Read the model definition and answer for the solid it produces. Units are mm, in the model's axes. Coordinates: 2 decimals unless noted, no trailing zeros. Write each loop counter-clockwise with the first axis right and the second up, starting at its lowest first coordinate (ties: lowest second). Pieces come first, ordered by that corner, then holes.
(1) Straight lines are drawn through the part: line 1 along Z through (x, y) = (2.65, 13.25); line 2 along Y through (x, z) = (2.35, -90.5); line 3 along Z through (x, y) = (1.6, 1.5). For each, find the intervals that lie inside material, in ascending order.
(2) The part is cut by section A-A, the plane y = 13.25. Determine the outline of the cut face in (x, z), and give its area (3 significant figures).
(3) The part is cut by section C-C, the plane z = -89.5. Determine the outline of the cut face in (x, y), and give its area (3 significant figures).
(4) The part is cut by section B-B, the plane x = 1.35. Determine the outline of the cut face in (y, z).
(5) Given pin 1 (0.9 mm diameter, centred on x = 2, z = -92.5, fed in from +Y); pin 2 (1.5 mm diameter, centred on x = 2, z = -123, fed in from -Y); pin 3 (1.5 mm diameter, centred on x = 1.5, y = 13.5, fed in from -Z), each flat-ended and moving along its own axis, determine where each tip first touches the part or whether it passes through.
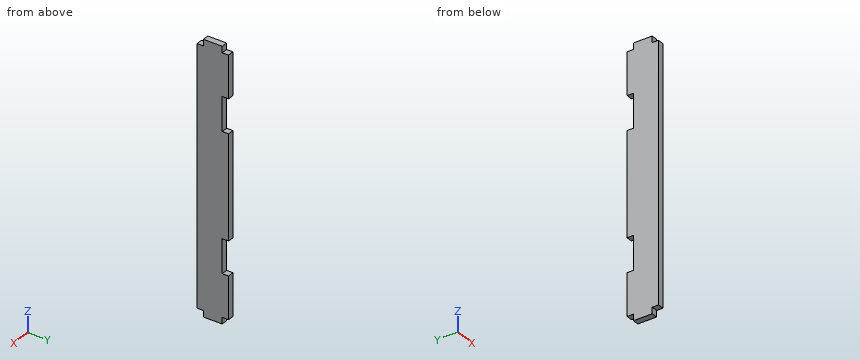
```python
from build123d import *

# Parameters (mm, degrees)
SKETCH1_W           = 3
SKETCH1_H           = 9
BOSS_EXTRUDE1_DEPTH = 3


with BuildPart() as part:
    # Sketch1 → Boss-Extrude1 (new body)
    with BuildSketch(Plane(origin=(0, 0, 0), x_dir=(0, 0, -1), z_dir=(1, 0, 0))):
        Polygon((0, 3), (0, 0), (121, 0), (121, 3), (121, 12), (121, 15), (101, 15), (101, 12), (85, 12), (85, 15), (36, 15), (36, 12), (20, 12), (20, 15), (0, 15), (0, 12), align=None)
        with Locations((-1.5, 7.5)):
            Rectangle(SKETCH1_W, SKETCH1_H)
        with Locations((122.5, 7.5)):
            Rectangle(SKETCH1_W, SKETCH1_H)
    extrude(amount=BOSS_EXTRUDE1_DEPTH)


solid = part.part
```
Computed:
1. line 1: z = -121 to -101, -85 to -36, -20 to 0
1. line 2: y = 0 to 12
1. line 3: z = -121 to 0
2. outline: (0, -121) - (3, -121) - (3, -101) - (0, -101) - close; (0, -85) - (3, -85) - (3, -36) - (0, -36) - close; (0, -20) - (3, -20) - (3, 0) - (0, 0) - close
2. area: 267 mm2
3. outline: (0, 0) - (3, 0) - (3, 12) - (0, 12) - close
3. area: 36.0 mm2
4. outline: (0, -121) - (3, -121) - (3, -124) - (12, -124) - (12, -121) - (15, -121) - (15, -101) - (12, -101) - (12, -85) - (15, -85) - (15, -36) - (12, -36) - (12, -20) - (15, -20) - (15, 0) - (12, 0) - (12, 3) - (3, 3) - (3, 0) - (0, 0) - close
5. pin 1: stops at y = 12
5. pin 2: stops at y = 3
5. pin 3: stops at z = -121
